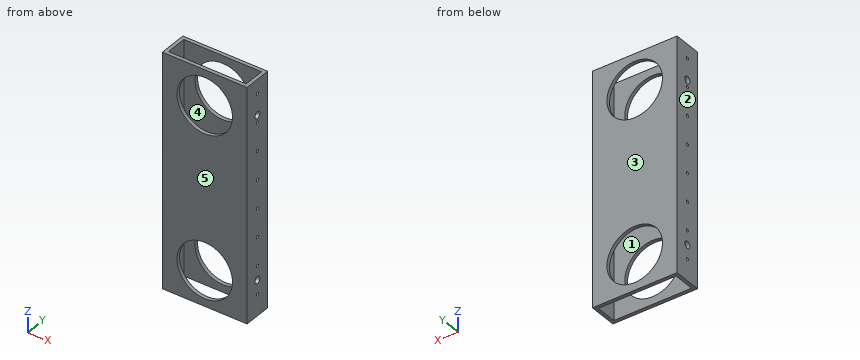
from build123d import *

# Parameters (mm, degrees)
SKETCH2_W           = 76.2
SKETCH2_H           = 25.4
SKETCH2_W_2         = 69.85
SKETCH2_H_2         = 19.05
EXTRUDE_THIN1_DEPTH = 209.55
SKETCH3_R           = 24.97201
CUT_EXTRUDE1_DEPTH  = 26.4
SKETCH4_R           = 1.3335
CUT_EXTRUDE2_DEPTH  = 77.2
LPATTERN1_COUNT     = 9
LPATTERN1_PITCH     = 25.4
SKETCH5_R           = 3.175
CUT_EXTRUDE3_DEPTH  = 77.2


with BuildPart() as part:
    # Sketch2 → Extrude-Thin1 (new body)
    with BuildSketch(Plane.XY):
        Rectangle(SKETCH2_W, SKETCH2_H)
        Rectangle(SKETCH2_W_2, SKETCH2_H_2, mode=Mode.SUBTRACT)
    extrude(amount=EXTRUDE_THIN1_DEPTH)

    # Sketch3 → Cut-Extrude1 (cut, through all)
    with BuildSketch(Plane(origin=(0, 12.7, 0), x_dir=(1, 0, 0), z_dir=(0, 1, 0))):
        with Locations((0, -177.8)):
            Circle(SKETCH3_R)
        with Locations((0, -31.75)):
            Circle(SKETCH3_R)
    extrude(amount=-CUT_EXTRUDE1_DEPTH, mode=Mode.SUBTRACT)

    # Sketch4 → Cut-Extrude2 (cut, through all)
    with BuildSketch(Plane(origin=(38.1, 0, 0), x_dir=(0, 0, -1), z_dir=(1, 0, 0))):
        with Locations((-196.85, 0)):
            Circle(SKETCH4_R)
    cut_extrude2 = extrude(amount=-CUT_EXTRUDE2_DEPTH, mode=Mode.SUBTRACT)

    # LPattern1: Cut-Extrude2 ×9
    with Locations(*[(0, 0, -i * LPATTERN1_PITCH) for i in range(1, LPATTERN1_COUNT)]):
        add(cut_extrude2, mode=Mode.SUBTRACT)

    # Sketch5 → Cut-Extrude3 (cut, through all)
    with BuildSketch(Plane(origin=(38.1, 0, 0), x_dir=(0, 0, -1), z_dir=(1, 0, 0))):
        with Locations((-31.75, 0)):
            Circle(SKETCH5_R)
        with Locations((-177.8, 0)):
            Circle(SKETCH5_R)
    extrude(amount=-CUT_EXTRUDE3_DEPTH, mode=Mode.SUBTRACT)


solid = part.part
Part model, mm, in its own coordinate system. Face numbers are marked on the shaded views. A direction names the side the tool comes from. Round coordinates to 2 decimals unless told otherwise and drop trailing zeros. Loops run counter-clockwise (first coordinate to the right, second up) from the corner with the lowest first, then second, coordinate; pieces in that order, holes last. Notation, with made-up numbers: (-16.5, 10) - (18.5, 10) arc R21 ccw to (18.5, 32) - close; hole circle Ø1 at (39, -13.75). An arc over 180 degrees is marked (long way). Answer as a JSON object with one key per item and string values.
Item 1: Band-saw the part on A-A on x = 30.5. List the corners of the cut face in (y, z) (3 decimals).
Output:
{"outline": "(-12.7, 0) - (-9.525, 0) - (-9.525, 209.55) - (-12.7, 209.55) - close; (9.525, 0) - (12.7, 0) - (12.7, 209.55) - (9.525, 209.55) - close"}
Item 2: Band-saw the part on C-C on x = 0. List the corners of the cut face in (y, z) (3 decimals).
Output:
{"outline": "(-12.7, 0) - (-9.525, 0) - (-9.525, 6.778) - (-12.7, 6.778) - close; (-12.7, 56.722) - (-9.525, 56.722) - (-9.525, 152.828) - (-12.7, 152.828) - close; (-12.7, 202.772) - (-9.525, 202.772) - (-9.525, 209.55) - (-12.7, 209.55) - close; (9.525, 0) - (12.7, 0) - (12.7, 6.778) - (9.525, 6.778) - close; (9.525, 56.722) - (12.7, 56.722) - (12.7, 152.828) - (9.525, 152.828) - close; (9.525, 202.772) - (12.7, 202.772) - (12.7, 209.55) - (9.525, 209.55) - close"}
Item 3: Band-saw the part on B-B on y = -7.25. List the corners of the cut face in (x, z) (3 decimals), plus the area to 3 significant figures.
Output:
{"outline": "(-38.1, 0) - (-34.925, 0) - (-34.925, 209.55) - (-38.1, 209.55) - close; (34.925, 0) - (38.1, 0) - (38.1, 209.55) - (34.925, 209.55) - close", "area": "1,330 mm2"}
Item 4: Pull direction X, two halves, no side cores. Call the marked faces 1, 2 and 3: pulls with the +X half, pulls with the -X half, needs draft (parallel to the pull), parting line crosses it, or undercut.
Output:
{"face 1": "undercut", "face 2": "pulls with the -X half", "face 3": "needs draft"}
Item 5: Wall check: L1, parallel to Z at x = 0, y = 11.7; L2, parallel to Y at x = 37.4, z = 177.8 (3 decimals); L3, parallel to Y at x = -36.7, z = 44.45. Give the ranges that are in metal, low to high.
Output:
{"L1": "0 to 6.78, 56.72 to 152.83, 202.77 to 209.55", "L2": "-12.7 to -3.175, 3.175 to 12.7", "L3": "-12.7 to -1.33, 1.33 to 12.7"}
Item 6: Tool access for the marked faces 4 and 5: list every direction of +Z, -Z, +X, -X, +Y, -Y with a clear straight run to the whole face (end or side of a thin tool).
Output:
{"face 4": "+Z, -Z", "face 5": "+Z, -Z, +X, -X, -Y"}
Item 7: Pin check, flat tip, straight feed: pin 1 (2.5 mm diameter, centred on y = 0, z = 95.25, fed in from -X). Stop position of the tip, or through.
Output:
{"pin 1": "through"}
Item 8: Band-saw the part on D-D on z = 83. List the corners of the cut face in (x, y) (3 decimals).
Output:
{"outline": "(-38.1, -12.7) - (38.1, -12.7) - (38.1, 12.7) - (-38.1, 12.7) - close; hole (-34.925, -9.525) - (34.925, -9.525) - (34.925, 9.525) - (-34.925, 9.525) - close"}
